```python
from build123d import *

# Parameters (mm, degrees)
BOSS_EXTRUDE1_DEPTH     = 95
BOSS_EXTRUDE2_DEPTH     = 25
BOSS_EXTRUDE3_DEPTH     = 35
CUT_EXTRUDE1_DEPTH      = 20
SKETCH4_R               = 38.333333333
SKETCH4_R_2             = 20.5
BOSS_EXTRUDE4_DEPTH     = 120
SKETCH5_R               = 35.5
SKETCH5_R_2             = 20.5
BOSS_EXTRUDE5_DEPTH     = 120
BOSS_EXTRUDE6_START     = 10
SKETCH6_R               = 35.5
SKETCH6_R_2             = 20.5
BOSS_EXTRUDE6_DEPTH     = 10
BOSS_EXTRUDE7_START     = 10
SKETCH7_R               = 38.333333333
SKETCH7_R_2             = 20.5
BOSS_EXTRUDE7_DEPTH     = 10
SKETCH8_R               = 20.5
CUT_EXTRUDE2_DEPTH      = 283.146731022
SKETCH9_R               = 20.5
CUT_EXTRUDE3_DEPTH      = 275.681684551
SKETCH10_R              = 15
CUT_EXTRUDE4_DEPTH      = 10
CUT_EXTRUDE5_DEPTH      = 194.412412161
CUT_EXTRUDE5_DEPTH_BACK = 194.412412161
SKETCH11_R              = 7.5
CHAMFER1_SIZE           = 2


with BuildPart() as part:
    # Sketch1 → Boss-Extrude1 (new body)
    with BuildSketch(Plane(origin=(0, 0, 0), x_dir=(1, 0, 0), z_dir=(0, 1, 0))):
        with BuildLine():
            Line((-70, -26.5), (-70, -106.5))
            Line((-70, -106.5), (-55, -106.5))
            Line((-55, -106.5), (-55, -40.423048454))
            ThreePointArc((-55, -40.423048454), (4.246212025, -10.746212025), (33.923048454, 48.5))
            Line((33.923048454, 48.5), (100, 48.5))
            Line((100, 48.5), (100, 63.5))
            Line((100, 63.5), (20, 63.5))
            ThreePointArc((20, 63.5), (-6.360389693, -0.139610307), (-70, -26.5))
        make_face()
    extrude(amount=BOSS_EXTRUDE1_DEPTH)

    # Sketch1_3 → Boss-Extrude2 (add)
    with BuildSketch(Plane(origin=(0, 0, 0), x_dir=(1, 0, 0), z_dir=(0, 1, 0))):
        with BuildLine():
            Line((-90, -106.5), (-70, -106.5))
            Line((-70, -106.5), (-70, -26.5))
            ThreePointArc((-70, -26.5), (-6.360389693, -0.139610307), (20, 63.5))
            Line((20, 63.5), (100, 63.5))
            Line((100, 63.5), (100, 96.5))
            ThreePointArc((100, 96.5), (97.071067812, 103.571067812), (90, 106.5))
            Line((90, 106.5), (-90, 106.5))
            ThreePointArc((-90, 106.5), (-97.071067812, 103.571067812), (-100, 96.5))
            Line((-100, 96.5), (-100, -96.5))
            ThreePointArc((-100, -96.5), (-97.071067812, -103.571067812), (-90, -106.5))
        make_face()
        with BuildLine():
            Line((-55, -40.423048454), (-55, -106.5))
            Line((-55, -106.5), (40, -106.5))
            Line((40, -106.5), (40, -56.5))
            ThreePointArc((40, -56.5), (42.928932188, -49.428932188), (50, -46.5))
            Line((50, -46.5), (100, -46.5))
            Line((100, -46.5), (100, 48.5))
            Line((100, 48.5), (33.923048454, 48.5))
            ThreePointArc((33.923048454, 48.5), (4.246212025, -10.746212025), (-55, -40.423048454))
        make_face()
    extrude(amount=BOSS_EXTRUDE2_DEPTH)

    # Sketch1_4 → Boss-Extrude3 (add)
    with BuildSketch(Plane(origin=(0, 0, 0), x_dir=(1, 0, 0), z_dir=(0, 1, 0))):
        with BuildLine():
            Line((40, -56.5), (40, -106.5))
            Line((40, -106.5), (90, -106.5))
            ThreePointArc((90, -106.5), (97.071067812, -103.571067812), (100, -96.5))
            Line((100, -96.5), (100, -46.5))
            Line((100, -46.5), (50, -46.5))
            ThreePointArc((50, -46.5), (42.928932188, -49.428932188), (40, -56.5))
        make_face()
    extrude(amount=BOSS_EXTRUDE3_DEPTH)

    # Sketch2 → Cut-Extrude1 (cut)
    with BuildSketch(Plane(origin=(0, 25, 0), x_dir=(1, 0, 0), z_dir=(0, 1, 0))):
        with BuildLine():
            Line((81, 39.5), (49.247641486, 39.5))
            ThreePointArc((49.247641486, 39.5), (43.223496519, 37.481834214), (39.630896205, 32.241935484))
            ThreePointArc((39.630896205, 32.241935484), (10.610173055, -17.110173055), (-38.741935484, -46.130896205))
            ThreePointArc((-38.741935484, -46.130896205), (-43.981834214, -49.723496519), (-46, -55.747641486))
            Line((-46, -55.747641486), (-46, -87.5))
            ThreePointArc((-46, -87.5), (-43.071067812, -94.571067812), (-36, -97.5))
            Line((-36, -97.5), (21, -97.5))
            ThreePointArc((21, -97.5), (28.071067812, -94.571067812), (31, -87.5))
            Line((31, -87.5), (31, -56.5))
            ThreePointArc((31, -56.5), (36.564971157, -43.064971157), (50, -37.5))
            Line((50, -37.5), (81, -37.5))
            ThreePointArc((81, -37.5), (88.071067812, -34.571067812), (91, -27.5))
            Line((91, -27.5), (91, 29.5))
            ThreePointArc((91, 29.5), (88.071067812, 36.571067812), (81, 39.5))
        make_face()
    extrude(amount=-CUT_EXTRUDE1_DEPTH, mode=Mode.SUBTRACT)

    # Sketch4 → Boss-Extrude4 (add)
    with BuildSketch(Plane(origin=(100, 0, 0), x_dir=(0, 0, -1), z_dir=(1, 0, 0))):
        with Locations((56, 95)):
            Circle(SKETCH4_R)
        with Locations((56, 95)):
            Circle(SKETCH4_R_2, mode=Mode.SUBTRACT)
    extrude(amount=-BOSS_EXTRUDE4_DEPTH)

    # Sketch5 → Boss-Extrude5 (add)
    with BuildSketch(Plane.XY.offset(106.5)):
        with Locations((-62.5, 95)):
            Circle(SKETCH5_R)
        with Locations((-62.5, 95)):
            Circle(SKETCH5_R_2, mode=Mode.SUBTRACT)
    extrude(amount=-BOSS_EXTRUDE5_DEPTH)

    # Sketch6 → Boss-Extrude6 (add)
    with BuildSketch(Plane.XY.offset(106.5).offset(BOSS_EXTRUDE6_START)):
        with Locations((-62.5, 95)):
            Circle(SKETCH6_R)
        with Locations((-62.5, 95)):
            Circle(SKETCH6_R_2, mode=Mode.SUBTRACT)
    extrude(amount=-BOSS_EXTRUDE6_DEPTH)

    # Sketch7 → Boss-Extrude7 (add)
    with BuildSketch(Plane(origin=(100, 0, 0), x_dir=(0, 0, -1), z_dir=(1, 0, 0)).offset(BOSS_EXTRUDE7_START)):
        with Locations((56, 95)):
            Circle(SKETCH7_R)
        with Locations((56, 95)):
            Circle(SKETCH7_R_2, mode=Mode.SUBTRACT)
    extrude(amount=-BOSS_EXTRUDE7_DEPTH)

    # Sketch8 → Cut-Extrude2 (cut, through all)
    with BuildSketch(Plane.XY.offset(116.5)):
        with Locations((-62.5, 95)):
            Circle(SKETCH8_R)
    extrude(amount=-CUT_EXTRUDE2_DEPTH, mode=Mode.SUBTRACT)

    # Sketch9 → Cut-Extrude3 (cut, through all)
    with BuildSketch(Plane(origin=(110, 0, 0), x_dir=(0, 0, -1), z_dir=(1, 0, 0))):
        with Locations((56, 95)):
            Circle(SKETCH9_R)
    extrude(amount=-CUT_EXTRUDE3_DEPTH, mode=Mode.SUBTRACT)

    # Sketch10 → Cut-Extrude4 (cut)
    with BuildSketch(Plane(origin=(0, 35, 0), x_dir=(1, 0, 0), z_dir=(0, 1, 0))):
        with Locations(Location((70, -76.5, 0), (0, 0, 270))):
            Circle(SKETCH10_R)
    extrude(amount=-CUT_EXTRUDE4_DEPTH, mode=Mode.SUBTRACT)

    # Sketch11 → Cut-Extrude5 (cut, two sides: drawn at the far end of the back side and taken through both)
    with BuildSketch(Plane(origin=(0, 25, 0), x_dir=(1, 0, 0), z_dir=(0, 1, 0)).offset(-CUT_EXTRUDE5_DEPTH_BACK)):
        with Locations(Location((70, -76.5, 0), (0, 0, 270))):
            Circle(SKETCH11_R)
    extrude(amount=CUT_EXTRUDE5_DEPTH + CUT_EXTRUDE5_DEPTH_BACK, mode=Mode.SUBTRACT)

    # Chamfer1
    chamfer1_edges = [part.edges().sort_by_distance(p)[0] for p in [
        (-20, 95, -35.5),
        (-83, 95, -13.5),
        (-83, 95, 116.5),
        (110, 95, -35.5),
    ]]
    chamfer(chamfer1_edges, length=CHAMFER1_SIZE)


solid = part.part
```
Read the model definition and answer for the solid it produces. Units are mm, in the model's axes. A direction names the side the tool comes from. Coordinates: 2 decimals unless noted, no trailing zeros. Order: outer loops, then holes, each group sorted by start corner. A loop starts at its lowest first (then second) coordinate and runs counter-clockwise, first axis right, second up. Notation, with made-up numbers: (58, -23.5) - (70, -23.5) arc R23 ccw to (70, -7.5) - close; hole circle Ø8 at (0, 3). An arc over 180 degrees is marked (long way). Answer as a JSON object with one key per item and string values. Group by question number.
Item 1: Flat-ended cylindrical pins translate along their axes: P1, Ø10, axis at y = 75.5, z = -33, coming from the -X side; P2, Ø8, axis at x = 58, z = 57, coming from the +Y side; P3, Ø1.5, axis at x = 68, z = -73, coming from the +Y side; P4, Ø9, axis at x = 70, z = 76.5, coming from the +Y side (3 decimals). Find the tip coordinate at first contact, or state that the pin passes through.
Item 2: Section D-D (z = -56) is taken. Give the vertices of the cut face in (x, y).
Item 3: The mould has two halves that part along Y. Classify faces 1 (the face through (65, 15, 37.5)), 2 (the face through (-24, 25, -49)), 3 (the face through (77, 25, 80)): +Y half, -Y half, draft (parallel to the pull), parting line (faces both ways), or undercut.
Item 4: A tool of negligible diameter and unlimited length cuts with its end or side. For faces 4 (the face through (-43.15, 15.14, 94.49)), 5 (the face through (-70, 42, 66)), 6 (the face through (-97.15, 12.32, 103.49)), 7 (the face through (-55, 42, 74)), from which of +Z, -Z, +X, -X, +Y, -Y can it reach the whole face along a straight path? Write none if from no direction.
Item 5: Section C-C (y = 13) is taken. Give the vertices of the cut face in (x, z).
Item 6: Section B-B (z = 76.5) is taken. Give the vertices of the cut face in (x, y).
Item 7: Section A-A (x = 70) is taken. Give the vertices of the cut face in (y, z).
Item 8: Consider probe 1 along X at (y, z) = (9, 76.5); probe 2 along Y at (x, z) = (-62.5, 34.5); probe 3 along Y at (x, z) = (61, -68). Determine where each line is inside the solid, lowest interval first. Write a range as from..to.
Results are:
{
 "1": {"P1": "stops at x = -20", "P2": "stops at y = 35", "P3": "stops at y = 129.72", "P4": "passes through"},
 "2": {"outline": "(-100, 0) - (100, 0) - (100, 56.67) - (110, 56.67) - (110, 72.5) - (108, 74.5) - (-18, 74.5) - (-20, 72.5) - (-20, 56.67) - (19.69, 56.67) - (19.69, 25) - (-100, 25) - close; (-20, 117.5) - (-18, 115.5) - (108, 115.5) - (110, 117.5) - (110, 133.33) - (-20, 133.33) - close"},
 "3": {"face 1": "draft", "face 2": "undercut", "face 3": "+Y half"},
 "4": {"face 4": "none", "face 5": "+Z, -Z, -X", "face 6": "+Z, -X, -Y", "face 7": "+Z"},
 "5": {"outline": "(-100, -96.5) arc R10 ccw to (-90, -106.5) - (90, -106.5) arc R10 ccw to (100, -96.5) - (100, 96.5) arc R10 ccw to (90, 106.5) - (-90, 106.5) arc R10 ccw to (-100, 96.5) - close; hole (-46, 55.75) arc R10 ccw to (-38.74, 46.13) arc R114 cw to (39.63, -32.24) arc R10 ccw to (49.25, -39.5) - (81, -39.5) arc R10 ccw to (91, -29.5) - (91, 27.5) arc R10 ccw to (81, 37.5) - (50, 37.5) arc R19 cw to (31, 56.5) - (31, 87.5) arc R10 ccw to (21, 97.5) - (-36, 97.5) arc R10 ccw to (-46, 87.5) - close; hole circle Ø15 at (70, 76.5)"},
 "6": {"outline": "(-100, 0) - (62.5, 0) - (62.5, 25) - (55, 25) - (55, 35) - (40, 35) - (40, 25) - (31, 25) - (31, 5) - (-46, 5) - (-46, 25) - (-55, 25) - (-55, 60.3) arc R35.5 ccw (long way) to (-70, 60.3) - (-70, 25) - (-100, 25) - close; (77.5, 0) - (100, 0) - (100, 35) - (85, 35) - (85, 25) - (77.5, 25) - close; hole circle Ø41 at (-62.5, 95)"},
 "7": {"outline": "(0, -106.5) - (25, -106.5) - (25, -63.5) - (57.41, -63.5) arc R38.33 ccw (long way) to (57.41, -48.5) - (25, -48.5) - (25, -39.5) - (5, -39.5) - (5, 37.5) - (25, 37.5) - (25, 46.5) - (35, 46.5) - (35, 61.5) - (25, 61.5) - (25, 69) - (0, 69) - close; (0, 84) - (25, 84) - (25, 91.5) - (35, 91.5) - (35, 106.5) - (0, 106.5) - close; hole circle Ø41 at (95, -56)"},
 "8": {"probe 1": "x = -100..-46, 31..62.5, 77.5..100", "probe 2": "y = 0..74.5, 115.5..130.5", "probe 3": "y = 0..25, 58.59..78.38, 111.62..131.41"}
}
